For this review, take the finished solid that the model builds, in its own axes (mm). Face numbers are marked on the shaded views. Give positions to 0.01 mm unless a question says otherwise; leave off trailing zeros. Order: outer loops, then holes, each group sorted by start corner. A loop starts at its lowest first (then second) coordinate and runs counter-clockwise, first axis right, second up.
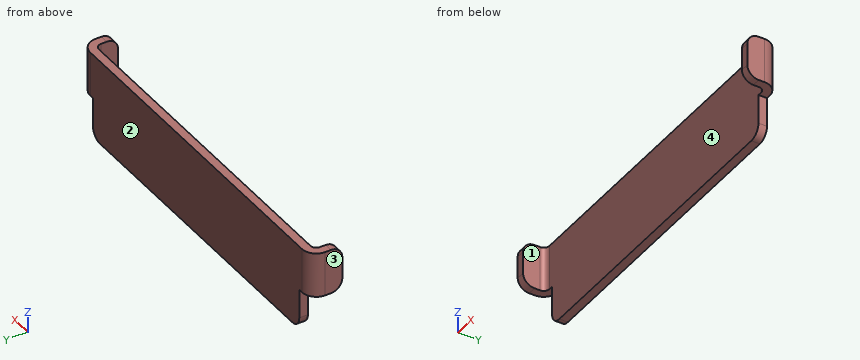
from build123d import *

# Parameters (mm, degrees)
SKETCH1_W                       = 64
SKETCH1_H                       = 15.060468003
BASE_FLANGE1_DEPTH              = 1.5
EDGE_FLANGE1_STRIP_W            = 8
EDGE_FLANGE1_STRIP_H            = 1.5
EDGE_FLANGE1_STRIP_CUT_DEPTH    = 7.904411042
EDGE_FLANGE1_RELIEF_W           = 8.75
EDGE_FLANGE1_RELIEF_H           = 0.75
EDGE_FLANGE1_RELIEF_CUT_DEPTH   = 1.5
EDGE_FLANGE1_STRIP_2_W          = 8
EDGE_FLANGE1_STRIP_2_H          = 1.5
EDGE_FLANGE1_STRIP_CUT_2_DEPTH  = 7.92099203
EDGE_FLANGE1_RELIEF_2_W         = 8.75
EDGE_FLANGE1_RELIEF_2_H         = 0.75
EDGE_FLANGE1_RELIEF_CUT_2_DEPTH = 1.5
EDGE_FLANGE1_DEPTH              = 7.904411042
EDGE_FLANGE1_BEND_DEPTH         = 7.92099203
SKETCH31_W                      = 3.25
SKETCH31_H                      = 6.406056961
SKETCH31_H_2                    = 6.389475973
CUT_EXTRUDE1_DEPTH              = 10
FILLET1_R                       = 2


# Sheet-metal steps are written as plain solids
with BuildPart() as part:
    # Sketch1 → Base-Flange1 (new body)
    with BuildSketch(Plane(origin=(0, 0, 0), x_dir=(1, 0, 0), z_dir=(0, 1, 0))):
        with Locations((32, 7.530234002)):
            Rectangle(SKETCH1_W, SKETCH1_H)
    extrude(amount=-BASE_FLANGE1_DEPTH)

    # Edge-Flange1 strip (across the edge) → Edge-Flange1 strip cut (cut)
    with BuildSketch(Plane(origin=(64, -1.5, -7.904411042), x_dir=(-1, 0, 0), z_dir=(0, 0, 1))):
        with Locations((-1.5, -0.75)):
            Rectangle(EDGE_FLANGE1_STRIP_W, EDGE_FLANGE1_STRIP_H)
    extrude(amount=EDGE_FLANGE1_STRIP_CUT_DEPTH, mode=Mode.SUBTRACT)

    # Edge-Flange1 relief (on the sheet) → Edge-Flange1 relief cut (cut)
    with BuildSketch(Plane(origin=(61.5, -1.5, -7.904411042), x_dir=(-1, 0, 0), z_dir=(0, -1, 0))):
        with Locations((-3.625, 0.375)):
            Rectangle(EDGE_FLANGE1_RELIEF_W, EDGE_FLANGE1_RELIEF_H)
    extrude(amount=-EDGE_FLANGE1_RELIEF_CUT_DEPTH, mode=Mode.SUBTRACT)

    # Edge-Flange1 strip 2 (across the edge) → Edge-Flange1 strip cut 2 (cut)
    with BuildSketch(Plane(origin=(0, -1.5, 0), x_dir=(1, 0, 0), z_dir=(0, 0, -1))):
        with Locations((-1.5, -0.75)):
            Rectangle(EDGE_FLANGE1_STRIP_2_W, EDGE_FLANGE1_STRIP_2_H)
    extrude(amount=EDGE_FLANGE1_STRIP_CUT_2_DEPTH, mode=Mode.SUBTRACT)

    # Edge-Flange1 relief 2 (on the sheet) → Edge-Flange1 relief cut 2 (cut)
    with BuildSketch(Plane(origin=(2.5, -1.5, 0), x_dir=(1, 0, 0), z_dir=(0, -1, 0))):
        with Locations((-3.625, -8.29599203)):
            Rectangle(EDGE_FLANGE1_RELIEF_2_W, EDGE_FLANGE1_RELIEF_2_H)
    extrude(amount=-EDGE_FLANGE1_RELIEF_CUT_2_DEPTH, mode=Mode.SUBTRACT)

    # Edge-Flange1 section (across the edge) → Edge-Flange1 (add)
    with BuildSketch(Plane(origin=(64, -1.5, -7.904411042), x_dir=(-1, 0, 0), z_dir=(0, 0, 1))):
        with BuildLine():
            Line((0, 1), (0, 4))
            Line((0, 4), (1.5, 4))
            Line((1.5, 4), (1.5, 1))
            ThreePointArc((1.5, 1), (1.792893219, 0.292893219), (2.5, 0))
            Line((2.5, 0), (2.5, -1.5))
            ThreePointArc((2.5, -1.5), (0.732233047, -0.767766953), (0, 1))
        make_face()
    extrude(amount=EDGE_FLANGE1_DEPTH)

    # Edge-Flange1 section 2 (across the edge) → Edge-Flange1 bend (add)
    with BuildSketch(Plane(origin=(0, -1.5, 0), x_dir=(1, 0, 0), z_dir=(0, 0, -1))):
        with BuildLine():
            Line((0, 1), (0, 4))
            Line((0, 4), (1.5, 4))
            Line((1.5, 4), (1.5, 1))
            ThreePointArc((1.5, 1), (1.792893219, 0.292893219), (2.5, 0))
            Line((2.5, 0), (2.5, -1.5))
            ThreePointArc((2.5, -1.5), (0.732233047, -0.767766953), (0, 1))
        make_face()
    extrude(amount=EDGE_FLANGE1_BEND_DEPTH)

    # Sketch31 → Cut-Extrude1 (cut)
    with BuildSketch(Plane(origin=(0, 0, 0), x_dir=(1, 0, 0), z_dir=(0, 1, 0))):
        with Locations((62.375, 11.857439523)):
            Rectangle(SKETCH31_W, SKETCH31_H)
        with Locations((1.625, 11.865730017)):
            Rectangle(SKETCH31_W, SKETCH31_H_2)
    extrude(amount=-CUT_EXTRUDE1_DEPTH, mode=Mode.SUBTRACT)

    # Fillet1
    fillet1_edges = [part.edges().sort_by_distance(p)[0] for p in [
        (60.75, -0.75, -15.060468003),
        (3.25, -0.75, -15.060468003),
        (63.25, -5.5, -7.904411042),
        (63.25, -5.5, 0),
        (0.75, -5.5, 0),
        (0.75, -5.5, -7.92099203),
    ]]
    fillet(fillet1_edges, radius=FILLET1_R)


solid = part.part
1) We need section C-C on x = 48. Give the boundary of the cut face in (y, z), then the cut area to 3 significant figures.
Answer sheet:
outline: (-1.5, -15.06) - (0, -15.06) - (0, 0) - (-1.5, 0) - close
area: 22.6 mm2
2) We need section A-A on y = -4.5. Give the boundary of the cut face in (x, z), then the cut area to 3 significant figures.
Answer sheet:
outline: (0, -7.65) - (1.5, -7.65) - (1.5, -0.27) - (0, -0.27) - close; (62.5, -7.64) - (64, -7.64) - (64, -0.27) - (62.5, -0.27) - close
area: 22.1 mm2
3) To check wall thickness, follow line 1 (X direction, y = -3.65, z = -1.75); line 2 (Y direction, x = 23.5, z = -8.25); line 3 (X direction, y = -0.5, z = -10.5). State the ranges of each line that lie inside material, in increasing order.
Answer sheet:
line 1: x = 0 to 1.5, 62.5 to 64
line 2: y = -1.5 to 0
line 3: x = 3.25 to 60.75
4) Clearance check with flat-ended pins moving along their axes: pin 1 (1 mm diameter, centred on x = 63, y = -1.5, fed in from -Z); pin 2 (3 mm diameter, centred on x = 40.5, z = -9.5, fed in from -Y); pin 3 (1.6 mm diameter, centred on y = -1, z = -10, fed in from -X). State where each tip first meets the part, or that it passes through.
Answer sheet:
pin 1: stops at z = -7.9
pin 2: stops at y = -1.5
pin 3: stops at x = 3.25
5) We need section B-B on z = -5. Give the boundary of the cut face in (x, y), then the cut area to 3 significant figures.
Answer sheet:
outline: (0, -5.5) - (1.5, -5.5) - (1.5, -2.5) arc R1 cw to (2.5, -1.5) - (61.5, -1.5) arc R1 cw to (62.5, -2.5) - (62.5, -5.5) - (64, -5.5) - (64, -2.5) arc R2.5 ccw to (61.5, 0) - (2.5, 0) arc R2.5 ccw to (0, -2.5) - close
area: 106 mm2
6) We need section D-D on z = -1. Give the boundary of the cut face in (x, y), then the cut area to 3 significant figures.
Answer sheet:
outline: (0, -5.23) - (1.5, -5.23) - (1.5, -2.5) arc R1 cw to (2.5, -1.5) - (61.5, -1.5) arc R1 cw to (62.5, -2.5) - (62.5, -5.23) - (64, -5.23) - (64, -2.5) arc R2.5 ccw to (61.5, 0) - (2.5, 0) arc R2.5 ccw to (0, -2.5) - close
area: 105 mm2
7) Draft analysis for pull direction X (two halves, no side actions). For the marked faces 1, 2, 3 and 4, state which applies: +X half, -X half, draft (parallel to the pull), parting line (faces both ways), or undercut.
Answer sheet:
face 1: undercut
face 2: draft
face 3: -X half
face 4: undercut
